Source: CAD feature listing. Evaluate the final solid. Frame: model axes, mm. Face numbers are marked on the shaded views. A direction names the side the tool comes from. Give positions to 0.01 mm unless a question says otherwise; leave off trailing zeros. Order: outer loops, then holes, each group sorted by start corner. A loop starts at its lowest first (then second) coordinate and runs counter-clockwise, first axis right, second up.
```python
from build123d import *

# Parameters (mm, degrees)
F2_SIZE  = 0.5
F3_R     = 5
F3_R_2   = 3.9
F4_DEPTH = 0.4
F5_R     = 2
F6_R     = 1.6
F7_DEPTH = 25
F8_R     = 3
F8_R_2   = 1.6
F9_DEPTH = 2.5


# Not quite as in the source:
# - a feature names something its author has since deleted; it is built from what else it names


with BuildPart() as f1:
    # F0 (on Front) → F1 (revolve)
    with BuildSketch(Plane.XZ):
        Polygon((3.9, 6), (0, 6), (0, 0), (10, 0), (10, 3), (3.9, 3), align=None)
    revolve(axis=Axis((0, 0, 3), (0, 0, -1)))

    # F2
    f2_edges = [f1.edges().sort_by_distance(p)[0] for p in [
        (-3.9, 0, 6),
    ]]
    chamfer(f2_edges, length=F2_SIZE)

    # F3 (on face) → F4 (join)
    with BuildSketch(Plane.XY.offset(3)):
        Circle(F3_R)
        Circle(F3_R_2, mode=Mode.SUBTRACT)
    extrude(amount=F4_DEPTH)

    # F5
    f5_edges = [f1.edges().sort_by_distance(p)[0] for p in [
        (-10, 0, 0),
    ]]
    fillet(f5_edges, radius=F5_R)

    # F6 (on face) → F7 (cut)
    with BuildSketch(Plane.XY.offset(6)):
        Circle(F6_R)
    extrude(amount=-F7_DEPTH, mode=Mode.SUBTRACT)

    # F8 (on face) → F9 (cut)
    with BuildSketch(Plane(origin=(0, 0, 0), x_dir=(1, 0, 0), z_dir=(0, 0, -1))):
        Circle(F8_R)
        Circle(F8_R_2, mode=Mode.SUBTRACT)
    extrude(amount=-F9_DEPTH, mode=Mode.SUBTRACT)


solid = f1.part
```
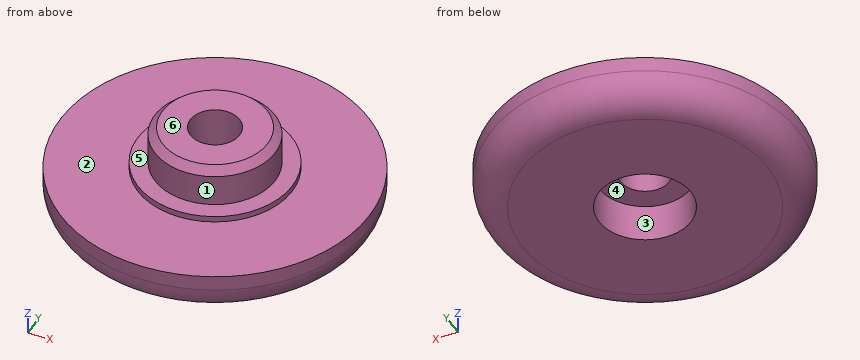
1) Material intervals for L1, parallel to Y at x = 0, z = 4.9; L2, parallel to Z at x = 3.75, y = -1.5; L3, parallel to Y at x = 0, z = 0.75, sorted ascending.
Report:
L1: y = -3.9 to -1.6, 1.6 to 3.9
L2: z = 0 to 3.4
L3: y = -9.56 to -3, 3 to 9.56
2) Section query C-C, the plane z = 4.35. Return the cut outline in (x, y).
Report:
outline: circle Ø7.8 at (0, 0); hole circle Ø3.2 at (0, 0)
3) Section query A-A, the plane x = 0. Return the cut outline in (y, z).
Report:
outline: (-10, 2) arc R2 ccw to (-8, 0) - (-3, 0) - (-3, 2.5) - (-1.6, 2.5) - (-1.6, 6) - (-3.4, 6) - (-3.9, 5.5) - (-3.9, 3.4) - (-5, 3.4) - (-5, 3) - (-10, 3) - close; (1.6, 2.5) - (3, 2.5) - (3, 0) - (8, 0) arc R2 ccw to (10, 2) - (10, 3) - (5, 3) - (5, 3.4) - (3.9, 3.4) - (3.9, 5.5) - (3.4, 6) - (1.6, 6) - close
4) Reachability of the marked faces 4, 5 and 6 from +Z, -Z, +X, -X, +Y, -Y: full face, straight path, thin tool, end or side. Return the list, or none.
Report:
face 4: -Z
face 5: +Z
face 6: +Z, +X, -X, +Y, -Y
5) Section query D-D, the plane z = 0.75. Return the cut outline in (x, y), and give its area (3 significant figures).
Report:
outline: circle Ø19.12 at (0, 0); hole circle Ø6 at (0, 0)
area: 259 mm2
6) Pin query (flat end, axial travel): pin 1 (1 mm diameter, centred on x = -4, z = 1, fed in from -Y); pin 2 (2 mm diameter, centred on y = -2.5, z = 3.5, fed in from +X); pin 3 (1 mm diameter, centred on x = -4, y = -5, fed in from +Z). Return the tip coordinate at first contact, or that it passes through.
Report:
pin 1: stops at y = -9.2
pin 2: stops at x = 9.87
pin 3: stops at z = 3
7) Draft query along X for the marked faces 1, 2 and 3. Return one class per face: +X half, -X half, draft (parallel to the pull), parting line (faces both ways), or undercut.
Report:
face 1: parting line
face 2: draft
face 3: undercut
